Read the model definition and answer for the solid it produces. Units are mm, in the model's axes. Face numbers are marked on the shaded views. A direction names the side the tool comes from. Coordinates: 2 decimals unless noted, no trailing zeros. Write item = value, one per line.
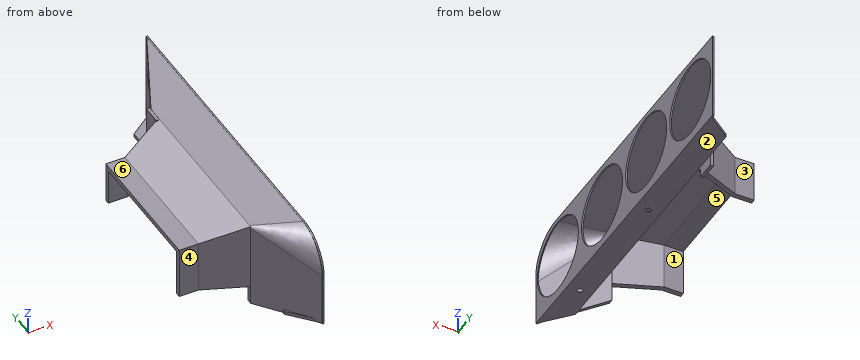
from build123d import *

# Parameters (mm, degrees)
PAD027_DEPTH    = 12
SKETCH076_R     = 1.75
PAD037_DEPTH    = 2
CHAMFER008_SIZE = 1.7
SKETCH098_R     = 24
PAD052_DEPTH    = 0.5
SKETCH099_W     = 11.665924
SKETCH099_H     = 40.921475
PAD053_DEPTH    = 2


with BuildPart() as part:
    # Sketch058 (on DatumPlane) → Pad027 (new body)
    with BuildSketch(Plane.YZ.offset(286)):
        Polygon((49, 12), (49, 45), (135, 45), (135, 19), (132, 19), (132, 42), (52, 42), (52, 12), align=None)
    extrude(amount=-PAD027_DEPTH)

    # Sketch060 (on DatumPlane) → AdditiveLoft001 section 0
    with BuildSketch(Plane.YZ.offset(313)):
        Polygon((41, 12), (41, 47), (143, 47), (143, 19), (146, 19), (146, 54.75), (38, 54.75), (38, 12), align=None)
    # Sketch059 (on DatumPlane) → AdditiveLoft001 section 1
    with BuildSketch(Plane.YZ.offset(286)):
        Polygon((49, 12), (49, 45), (135, 45), (135, 19), (132, 19), (132, 42), (52, 42), (52, 12), align=None)
    loft()

    # Sketch062 (on DatumPlane) → AdditiveLoft002 section 0
    with BuildSketch(Plane.YZ.offset(340)):
        with BuildLine():
            Line((3.2, 0), (3.2, 33.75))
            ThreePointArc((26.2, 56.75), (9.936544, 50.013456), (3.2, 33.75))
            Line((26.2, 56.75), (187, 56.75))
            Line((210, 56.75), (187, 56.75))
            Line((210, 54), (210, 56.75))
            Line((183, 54), (210, 54))
            Line((183, 54), (30, 54))
            ThreePointArc((30, 54), (12.32233, 46.67767), (5, 29))
            Line((5, 29), (5, 0))
            Line((5, 0), (3.2, 0))
        make_face()
    # Sketch061 (on DatumPlane) → AdditiveLoft002 section 1
    with BuildSketch(Plane.YZ.offset(313)):
        with BuildLine():
            Line((41, 0), (41, 45.742159))
            ThreePointArc((42.257841, 47), (41.368413, 46.631587), (41, 45.742159))
            Line((42.257841, 47), (141.742159, 47))
            Line((141.742159, 47), (154.714584, 47))
            Line((154.714584, 47), (154.714584, 54.75))
            Line((154.714584, 54.75), (144.742159, 54.75))
            Line((144.742159, 54.75), (39.257841, 54.75))
            ThreePointArc((39.257841, 54.75), (38.368413, 54.381587), (38, 53.492159))
            Line((38, 53.492159), (38, 0))
            Line((38, 0), (41, 0))
        make_face()
    loft()

    # Sketch076 → Pad037 (join)
    with BuildSketch(Plane.XY):
        Polygon((340, 208), (340, 3.768617), (325, 20.549414), (325, 196.984344), align=None)
        with Locations((332.5, 40)):
            Circle(SKETCH076_R, mode=Mode.SUBTRACT)
        with Locations((332.5, 120)):
            Circle(SKETCH076_R, mode=Mode.SUBTRACT)
    extrude(amount=PAD037_DEPTH)

    # Chamfer008
    chamfer008_edges = [part.edges().sort_by_distance(p)[0] for p in [
        (330.75, 120, 2),
        (330.75, 40, 2),
    ]]
    chamfer(chamfer008_edges, length=CHAMFER008_SIZE)

    # Sketch098 (on DatumPlane) → Pad052 (join, symmetric)
    with BuildSketch(Plane.YZ.offset(340)):
        with BuildLine():
            Line((3.2, 0), (3.2, 33.75))
            ThreePointArc((26.2, 56.75), (9.936544, 50.013456), (3.2, 33.75))
            Line((26.2, 56.75), (209.995, 56.75))
            ThreePointArc((210, 56.745), (209.998536, 56.748536), (209.995, 56.75))
            Line((210, 56.745), (210, 0))
            Line((210, 0), (208, 0))
            Line((5, 0), (208, 0))
            Line((5, 0), (3.2, 0))
        make_face()
        with Locations((29, 30)):
            Circle(SKETCH098_R, mode=Mode.SUBTRACT)
        with Locations((184, 30)):
            Circle(SKETCH098_R, mode=Mode.SUBTRACT)
        with Locations((80.663441, 29)):
            Circle(SKETCH098_R, mode=Mode.SUBTRACT)
        with Locations((132.326882, 30)):
            Circle(SKETCH098_R, mode=Mode.SUBTRACT)
    extrude(amount=PAD052_DEPTH, both=True)

    # Sketch099 (on DatumPlane) → Pad053 (join)
    with BuildSketch(Plane.YZ.offset(313)):
        with Locations((150.516098, 34.194787)):
            Rectangle(SKETCH099_W, SKETCH099_H)
    extrude(amount=-PAD053_DEPTH)


solid = part.part
1) Straight lines are drawn through the part: line 1 along Y through (x, z) = (340, 30); line 2 along Z through (x, y) = (339.95, 29); line 3 along X through (y, z) = (21, 6.5). For each, find the intervals that lie inside material, in ascending order. Write a range as from..to.
Returned:
line_1 = 3.2..5, 53..56.68, 104.64..108.33, 156.33..160, 208..210
line_2 = 0..6, 53.97..56.75
line_3 = 326.19..328, 339.5..340.5
2) The part is cut by section A-A (z = 21.5). Count the separate pieces of the cut face and the enclosed holes in it, and give its area (3 significant figures).
Returned:
separate_pieces = 6
enclosed_holes = 0
area = 346 mm^2
3) For the marked faces 1 and 2, determine the directions among +Z, -Z, +X, -X, +Y, -Y from which every point of the face is accessible in a straight line to the end or side of a thin tool.
Returned:
face_1 = -Z, -X
face_2 = -Z, +X, -X, +Y, -Y
4) Determine the mould class of the marked faces 3, 4, 5 and 6 for opening direction Y: pulls with the +Y half, pulls with the -Y half, needs draft (parallel to the pull), parting line crosses it, or undercut.
Returned:
face_3 = pulls with the +Y half
face_4 = pulls with the -Y half
face_5 = undercut
face_6 = needs draft
5) Flat-ended cylindrical pins translate along their axes: pin 1 Ø0.6 at (y, z) = (41.5, 46.5) entering from -X; pin 2 Ø1.5 at (x, z) = (329.5, 47.5) entering from -Y; pin 3 Ø6 at (x, y) = (324, 137) entering from +Z; pin 4 Ø10 at (y, z) = (65.5, 17) entering from +X. Find the tip coordinate at first contact, or state that the pin passes through.
Returned:
pin_1 = 303.67
pin_2 = 17.21
pin_3 = 55.79
pin_4 = 340.5
